Source: CAD feature listing. Evaluate the final solid. Frame: model axes, mm. Face numbers are marked on the shaded views. Coordinates: 2 decimals unless noted, no trailing zeros. Write each loop counter-clockwise with the first axis right and the second up, starting at its lowest first coordinate (ties: lowest second). Pieces come first, ordered by that corner, then holes. Notation, with made-up numbers: M 74.5,67.25 L 113.5,67.25 A16 cw 113.5,98.25 Z; hole C 83,-18 d6. An arc over 180 degrees is marked long. One line per item, written item: value. Start each with the question number.
Item 1: Cut plane A-A, the plane x = -6. Output: boundary loops of the cut face in (y, z), then the cut area to 3 significant figures.
Item 2: Cut plane D-D, the plane z = 1.1. State how many separate pieces and enclosed holes the cut face has, then the cut area to 3 significant figures.
Item 3: Cut plane B-B, the plane y = 0. Output: boundary loops of the cut face in (x, z), then the cut area to 3 significant figures.
Item 4: Pin query (flat end, axial travel): P1, Ø3.5, axis at x = -43.99, y = -2.91, coming from the +Z side; P2, Ø2.5, axis at x = -42.51, y = 5.46, coming from the -Z side. Return the tip coordinate at first contact, or that it passes through.
Item 5: Mould query, pull axis Y, two halves, no side actions, for the marked faces 1, 2 and 3. Classes: released by +Y, released by -Y, zero draft, split by the parting line, or undercut.
Item 6: Cut plane C-C, the plane x = -18. Output: boundary loops of the cut face in (y, z).
Item 7: Ray query, L1, parallel to X at y = 2, z = 2.6; L2, parallel to X at y = -5, z = 3.1; L3, parallel to X at y = 9.5, z = 2.2. Return the intervals inside material, ascending. Write a range as from..to.
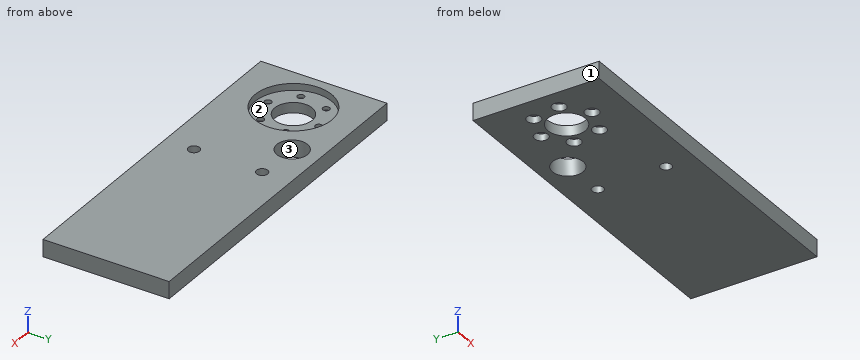
```python
from build123d import *

# Parameters (mm, degrees)
F0_W           = 100
F0_H           = 37
F1_DEPTH       = 5
F2_R           = 5.5
F3_DEPTH       = 5
F4_R           = 11.25
F5_DEPTH       = 2
F7_D           = 2
F7_DEPTH       = 6
F7_CBORE_D     = 4
F7_CBORE_DEPTH = 2
F7_TIP         = 0.600860619
F9_D           = 9
F9_DEPTH       = 7
F9_TIP         = 2.7038727856
F11_D          = 3.3
F11_DEPTH      = 6
F11_TIP        = 0.9914200214


with BuildPart() as f1:
    # F0 (on Top) → F1 (new body)
    with BuildSketch(Plane.XY):
        Rectangle(F0_W, F0_H)
    extrude(amount=F1_DEPTH)

    # F2 (on face) → F3 (cut)
    with BuildSketch(Plane.XY.offset(5)):
        with Locations((-36, 0)):
            Circle(F2_R)
    extrude(amount=-F3_DEPTH, mode=Mode.SUBTRACT)

    # F4 (on face) → F5 (cut)
    with BuildSketch(Plane.XY.offset(5)):
        with Locations((-36, 0)):
            Circle(F4_R)
    extrude(amount=-F5_DEPTH, mode=Mode.SUBTRACT)

    # F7
    with Locations(Plane(origin=(0, 0, 0), x_dir=(1, 0, 0), z_dir=(0, 0, -1))):
        with Locations((-37.4760095102, 8.3708659006), (-43.9873872767, 2.9071712183), (-42.5113777665, -5.4636946823), (-34.5239904898, -8.3708659006), (-28.0126127233, -2.9071712183), (-29.4886222335, 5.4636946823)):
            CounterBoreHole(F7_D / 2, F7_CBORE_D / 2, F7_CBORE_DEPTH, depth=F7_DEPTH)
            with Locations((0, 0, -(F7_DEPTH + F7_TIP / 2))):  # 118° drill point
                Cone(0, F7_D / 2, F7_TIP, mode=Mode.SUBTRACT)

    # F9
    with Locations(Plane.XY.offset(5)):
        with Locations((-19, 10.5)):
            Hole(F9_D / 2, depth=F9_DEPTH)
            with Locations((0, 0, -(F9_DEPTH + F9_TIP / 2))):  # 118° drill point
                Cone(0, F9_D / 2, F9_TIP, mode=Mode.SUBTRACT)

    # F11
    with Locations(Plane(origin=(0, 0, 0), x_dir=(1, 0, 0), z_dir=(0, 0, -1))):
        with Locations((-6, 10), (-6, -10)):
            Hole(F11_D / 2, depth=F11_DEPTH)
            with Locations((0, 0, -(F11_DEPTH + F11_TIP / 2))):  # 118° drill point
                Cone(0, F11_D / 2, F11_TIP, mode=Mode.SUBTRACT)


solid = f1.part
```
From the geometry:
1. outline: M -18.5,0 L -11.65,0 L -11.65,5 L -18.5,5 Z; M -8.35,0 L 8.35,0 L 8.35,5 L -8.35,5 Z; M 11.65,0 L 18.5,0 L 18.5,5 L 11.65,5 Z
1. area: 152 mm²
2. separate pieces: 1
2. enclosed holes: 10
2. area: 3,450 mm²
3. outline: M -50,0 L -41.5,0 L -41.5,3 L -47.25,3 L -47.25,5 L -50,5 Z; M -30.5,0 L 50,0 L 50,5 L -24.75,5 L -24.75,3 L -30.5,3 Z
3. area: 422 mm²
4. P1: stops at z = 3
4. P2: stops at z = 2
5. face 1: zero draft
5. face 2: undercut
5. face 3: undercut
6. outline: M -18.5,0 L 6.11,0 L 6.11,5 L -18.5,5 Z; M 14.89,0 L 18.5,0 L 18.5,5 L 14.89,5 Z
7. L1: x = -50..-41.12, -30.88..-28.43, -27.59..50
7. L2: x = -50..-46.08, -25.92..50
7. L3: x = -50..-23.39, -14.61..-7.57, -4.43..50
